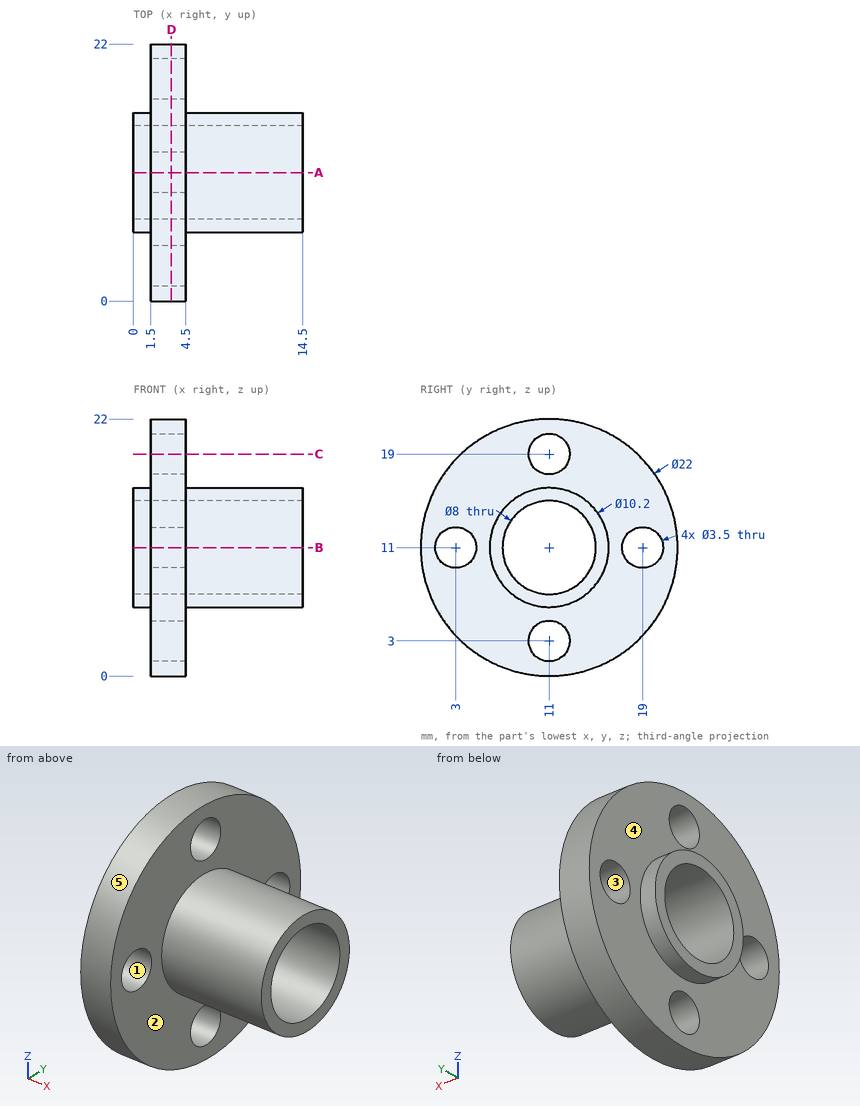
Drawing for the job (mm, zero at the part's lowest x, y, z). A direction names the side the tool comes from. Give positions to 0.01 mm unless a question says otherwise; leave off trailing zeros. Loops run counter-clockwise (first coordinate to the right, second up) from the corner with the lowest first, then second, coordinate; pieces in that order, holes last. Notation, with made-up numbers: M 47.5,-30 L 61.5,-30 A10 ccw 61.5,-17 Z; hole C -25.5,89 d4. An arc over 180 degrees is marked long. Use one line per item in the form item = value.
Item 1: Drill centre lines: probe 1 along Y at (x, z) = (2.7, 11); probe 2 along X at (y, z) = (21, 14.5); probe 3 along Z at (x, y) = (7.25, 14). Where is each one in solid material? Low to high. Write a range as from..to.
Determined:
probe_1 = 0..1.25, 4.75..7, 15..17.25, 20.75..22
probe_2 = 1.5..4.5
probe_3 = 6.88..8.35, 13.65..15.12
Item 2: Two-plate mould, pull along Z, no slides. Class the marked faces 3, 4 and 5: pulls with the +Z half, pulls with the -Z half, needs draft (parallel to the pull), parting line crosses it, or undercut.
Determined:
face_3 = undercut
face_4 = needs draft
face_5 = parting line crosses it
Item 3: Slice it at D-D (x = 3.25). List the corners of the cut face in (y, z).
Determined:
outline = C 11,11 d22; hole C 3,11 d3.5; hole C 11,11 d8; hole C 11,3 d3.5; hole C 11,19 d3.5; hole C 19,11 d3.5
Item 4: Flat gauge pins, fed straight in: pin 1 (5 mm diameter, centred on x = 12.5, y = 13, fed in from -Z); pin 2 (4 mm diameter, centred on y = 19, z = 11, fed in from +X); pin 3 (5.5 mm diameter, centred on y = 11, z = 3, fed in from -X); pin 4 (11 mm diameter, centred on y = 13, z = 10, fed in from -X). Where does each tip first touch, or does it go through?
Determined:
pin_1 = 5.9
pin_2 = 4.5
pin_3 = 1.5
pin_4 = 0
Item 5: Slice it at C-C (z = 19). List the corners of the cut face in (x, y).
Determined:
outline = M 1.5,3.45 L 4.5,3.45 L 4.5,9.25 L 1.5,9.25 Z; M 1.5,12.75 L 4.5,12.75 L 4.5,18.55 L 1.5,18.55 Z
Item 6: Slice it at A-A (y = 11). List the corners of the cut face in (x, z).
Determined:
outline = M 0,5.9 L 1.5,5.9 L 1.5,4.75 L 4.5,4.75 L 4.5,5.9 L 14.5,5.9 L 14.5,7 L 0,7 Z; M 0,15 L 14.5,15 L 14.5,16.1 L 4.5,16.1 L 4.5,17.25 L 1.5,17.25 L 1.5,16.1 L 0,16.1 Z; M 1.5,0 L 4.5,0 L 4.5,1.25 L 1.5,1.25 Z; M 1.5,20.75 L 4.5,20.75 L 4.5,22 L 1.5,22 Z
Item 7: Which spindle directions (+Z, -Z, +X, -X, +Y, -Y) get a long thin tool onto all of the face, cutting with end or side? Do the marked faces 1 and 2. Say none if no direction does.
Determined:
face_1 = +X, -X
face_2 = +X
